Geometry: final body of the model. Coordinates: model frame, mm. Face numbers are marked on the shaded views. A direction names the side the tool comes from. Give positions to 0.01 mm unless a question says otherwise; leave off trailing zeros. Order: outer loops, then holes, each group sorted by start corner. A loop starts at its lowest first (then second) coordinate and runs counter-clockwise, first axis right, second up. Notation, with made-up numbers: (72.5, 11.25) - (94.5, 11.25) arc R25 cw to (94.5, 34.25) - close; hole circle Ø9 at (36, 75.25). An arc over 180 degrees is marked (long way). Write item = value, one per line. Start each with the question number.
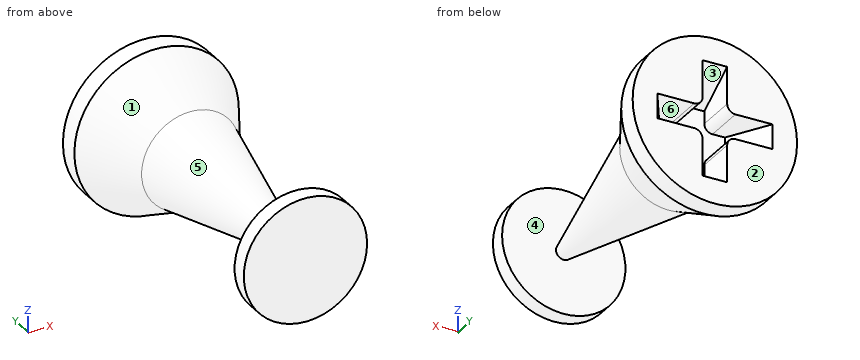
from build123d import *

# Parameters (mm, degrees)
F0_W      = 25.4
F0_H      = 25.4
F2_SIZE2  = 19.05
F2_SIZE   = 10.16
F3_W      = 7.62
F3_H      = 6.35
F3_W_2    = 6.35
F3_H_2    = 7.62
F4_DEPTH  = 12.7
F5_SIZE2  = 12.69999
F5_SIZE   = 7.61999
F6_R      = 2.54
F7_R      = 15.24
F8_DEPTH  = 63.5
F9_SIZE2  = 63.49999
F9_SIZE   = 13.96999
F10_R     = 19.05
F10_R_2   = 1.27001
F11_DEPTH = 5.08


# Not quite as in the source:
# - a fillet or chamfer is up to 0.001 mm smaller than in the source, because OpenCascade refuses the exact size


with BuildPart() as f1:
    # F0 (on Top) → F1 (revolve)
    with BuildSketch(Plane.XY):
        Rectangle(F0_W, F0_H)
    revolve(axis=Axis((-12.7, 0, 0), (0, 1, 0)))

    # F2
    f2_edges = [f1.edges().sort_by_distance(p)[0] for p in [
        (-38.1, -12.7, 0),
    ]]
    chamfer(f2_edges, length=F2_SIZE, length2=F2_SIZE2)

    # F3 (on face) → F4 (cut, symmetric)
    with BuildSketch(Plane(origin=(0, 12.7, 0), x_dir=(-1, 0, 0), z_dir=(0, 1, 0))):
        with Locations((12.7, 6.985)):
            Rectangle(F3_W, F3_H)
        with Locations((5.715, 0)):
            Rectangle(F3_W_2, F3_H_2)
        with Locations((12.7, 0)):
            Rectangle(F3_W, F3_H_2)
        with Locations((19.685, 0)):
            Rectangle(F3_W_2, F3_H_2)
        with Locations((12.7, -6.985)):
            Rectangle(F3_W, F3_H)
    extrude(amount=F4_DEPTH, both=True, mode=Mode.SUBTRACT)

    # F5 (size 7.62 and 12.7 in the source; OpenCascade refuses exactly that, so slightly less here)
    f5_edges = [f1.edges().sort_by_distance(p)[0] for p in [
        (-12.7, 12.7, 10.16),
        (-2.54, 12.7, 0),
        (-22.86, 12.7, 0),
        (-12.7, 12.7, -10.16),
    ]]
    chamfer(f5_edges, length=F5_SIZE, length2=F5_SIZE2)

    # F6
    f6_edges = [f1.edges().sort_by_distance(p)[0] for p in [
        (-8.89, 6.35, -3.81),
        (-16.51, 6.35, -3.81),
        (-8.89, 6.35, 3.81),
        (-16.51, 6.35, 3.81),
    ]]
    fillet(f6_edges, radius=F6_R)

    # F7 (on face) → F8 (join)
    with BuildSketch(Plane.XZ.offset(12.7)):
        with Locations((-12.7, 0)):
            Circle(F7_R)
    extrude(amount=F8_DEPTH)

    # F9 (size 13.97 and 63.5 in the source; OpenCascade refuses exactly that, so slightly less here)
    f9_edges = [f1.edges().sort_by_distance(p)[0] for p in [
        (-27.94, -76.2, 0),
    ]]
    f9_side = f1.faces().sort_by_distance((-12.7, -76.2, 0))[0]
    chamfer(f9_edges, length=F9_SIZE, length2=F9_SIZE2, reference=f9_side)

    # F10 (on face) → F11 (join)
    with BuildSketch(Plane.XZ.offset(76.2)):
        with Locations((-12.7, 0)):
            Circle(F10_R)
        with Locations((-12.7, 0)):
            Circle(F10_R_2, mode=Mode.SUBTRACT)
    extrude(amount=-F11_DEPTH)


solid = f1.part
Q1. Contact query for flat-ended pins moving along their axis: pin 1 (3 mm diameter, centred on y = -50, z = -4.5, fed in from +X); pin 2 (3.5 mm diameter, centred on x = -23, y = 8, fed in from +Z); pin 3 (1 mm diameter, centred on x = -6.5, y = -46.5, fed in from +Z). Output: stop coordinate, or through.
Q2. Section C-C, the plane y = -35. Return the cut outline in (x, z), then the cut area to 3 significant figures.
Q3. Section D-D, the plane y = -11. Return the cut outline in (x, z), then the cut area to 3 significant figures.
Q4. Material intervals for line 1 along Y through (x, z) = (3.5, -6); line 2 along Y through (x, z) = (2, 9.5); line 3 along Z through (x, y) = (-28, -9.5), sorted ascending. Write a range as from..to.
Q5. Set-up query: the marked faces 1, 2 and 3. Return all of +Z, -Z, +X, -X, +Y, -Y with unobstructed straight access to the full face (end or side cutting, diameter ignored); none if empty.
Q6. Pull-direction query (Z, two-part tool) for the marked faces 4, 5 and 6; classes: +Z half, -Z half, draft (parallel to the pull), parting line (faces both ways), or undercut.
The answers:
q1.pin_1 = -6.25
q1.pin_2 = 23.92
q1.pin_3 = 5.35
q2.outline = circle Ø20.67 at (-12.7, 0)
q2.area = 335 mm²
q3.outline = circle Ø32.29 at (-12.7, 0)
q3.area = 819 mm²
q4.line_1 = -76.2..-71.12, -8.88..12.7
q4.line_2 = -76.2..-71.12, -8.46..12.7
q4.line_3 = -7.29..7.29
q5.face_1 = none
q5.face_2 = +Z, -Z, +X, -X, +Y
q5.face_3 = +Y
q6.face_4 = draft
q6.face_5 = parting line
q6.face_6 = undercut
